```python
from build123d import *

# Parameters (mm, degrees)
SKETCH1_W           = 24
SKETCH1_H           = 3
BOSS_EXTRUDE1_DEPTH = 2
BOSS_EXTRUDE2_DEPTH = 3
BOSS_EXTRUDE3_DEPTH = 3
CUT_EXTRUDE1_REACH  = 23.383
SKETCH6_R           = 0.5
SKETCH9_W           = 3
SKETCH9_H           = 3
BOSS_EXTRUDE4_DEPTH = 0.5


with BuildPart() as part:
    # Sketch1 → Boss-Extrude1 (new body)
    with BuildSketch(Plane(origin=(0, 0, 0), x_dir=(1, 0, 0), z_dir=(0, 1, 0))):
        Rectangle(SKETCH1_W, SKETCH1_H)
    extrude(amount=BOSS_EXTRUDE1_DEPTH)

    # Sketch4 → Boss-Extrude2 (add)
    with BuildSketch(Plane(origin=(12, 0, 0), x_dir=(0, 0, -1), z_dir=(1, 0, 0))):
        Polygon((-11.5, 10), (-1.5, 0), (1.5, 0), (1.5, 2), (-0.5, 2), (-8.5, 10), align=None)
    extrude(amount=BOSS_EXTRUDE2_DEPTH)

    # Sketch5 → Boss-Extrude3 (add)
    with BuildSketch(Plane.ZY.offset(12)):
        Polygon((1.5, 0), (11.5, 10), (8.5, 10), (0.5, 2), (-1.5, 2), (-1.5, 0), align=None)
    extrude(amount=BOSS_EXTRUDE3_DEPTH)

    # Sketch6 → Cut-Extrude1 (cut, up to next)
    with BuildSketch(Plane.XZ, mode=Mode.PRIVATE) as cut_extrude1_sk1:
        with Locations(Location((-10, 0, 0), (0, 0, 270))):
            Circle(SKETCH6_R)
    cut_extrude1_tool1 = extrude(cut_extrude1_sk1.sketch, amount=-CUT_EXTRUDE1_REACH, mode=Mode.PRIVATE) & part.part
    # Sketch6 → Cut-Extrude1 (cut, up to next)
    with BuildSketch(Plane.XZ, mode=Mode.PRIVATE) as cut_extrude1_sk2:
        with Locations(Location((10, 0, 0), (0, 0, 270))):
            Circle(SKETCH6_R)
    cut_extrude1_tool2 = extrude(cut_extrude1_sk2.sketch, amount=-CUT_EXTRUDE1_REACH, mode=Mode.PRIVATE) & part.part
    add(cut_extrude1_tool1.solids().sort_by_distance((-10, 0, 0))[0], mode=Mode.SUBTRACT)
    add(cut_extrude1_tool2.solids().sort_by_distance((10, 0, 0))[0], mode=Mode.SUBTRACT)

    # Sketch9 → Boss-Extrude4 (add)
    with BuildSketch(Plane(origin=(0, 10, 0), x_dir=(1, 0, 0), z_dir=(0, 1, 0))):
        with Locations((-13.5, -10)):
            Rectangle(SKETCH9_W, SKETCH9_H)
        with Locations((13.5, -10)):
            Rectangle(SKETCH9_W, SKETCH9_H)
    extrude(amount=BOSS_EXTRUDE4_DEPTH)


solid = part.part
```
Input: part model. Units: mm. Frame: model coordinates. A direction names the side the tool comes from. Coordinates: 2 decimals unless noted, no trailing zeros. Loops run counter-clockwise (first coordinate to the right, second up) from the corner with the lowest first, then second, coordinate; pieces in that order, holes last. Notation, with made-up numbers: M 56,-30.75 L 114,-30.75 A27 cw 114,-8.75 Z; hole C 28,42 d4. An arc over 180 degrees is marked long. Use a Markdown table: item, result. Add a question column.
1) Section C-C, the plane z = 0. Return the cut outline in (x, y), plus the area to 3 significant figures.
2) Section B-B, the plane z = 4.75. Return the cut outline in (x, y), plus the area to 3 significant figures.
3) Draft query along X for faces 4 (the flat face through (0, 1, -1.5)), 5 (the flat face through (12, 6, 6)), 6 (the flat face through (-15, 5, 5)). Return one class per face: +X half, -X half, draft (parallel to the pull), parting line (faces both ways), or undercut.
4) Section A-A, the plane x = -10. Return the cut outline in (y, z).
5) Pin query (flat end, axial travel): P1, Ø0.9, axis at x = 3, z = 0.5, coming from the +Y side; P2, Ø1.6, axis at x = 2.5, y = 1, coming from the +Z side; P3, Ø3, axis at x = 0, z = 3.5, coming from the +Y side. Return the tip coordinate at first contact, or that it passes through.
6) Section D-D, the plane x = -0.5. Return the cut outline in (y, z).
7) Set-up query: faces 1 (the flat face through (0, 2, 0)), 2 (the flat face through (0, 1, 1.5)), 3 (the flat face through (15, 5, 5)). Return all of +Z, -Z, +X, -X, +Y, -Y with unobstructed straight access to the full face (end or side cutting, diameter ignored); none if empty.
8) Line query: L1, parallel to X at y = 0.85, z = 0; L2, parallel to X at y = 9.25, z = 8.25; L3, parallel to Y at x = -4.75, z = 0. Output: solid intervals per line, ascending. Write a range as from..to.
Answer below:
| question | item | result |
|---|---|---|
| 1 | outline | M -15,0 L -10.5,0 L -10.5,2 L -15,2 Z; M -9.5,0 L 9.5,0 L 9.5,2 L -9.5,2 Z; M 10.5,0 L 15,0 L 15,2 L 10.5,2 Z |
| 1 | area | 56.0 mm2 |
| 2 | outline | M -15,3.25 L -12,3.25 L -12,6.25 L -15,6.25 Z; M 12,3.25 L 15,3.25 L 15,6.25 L 12,6.25 Z |
| 2 | area | 18.0 mm2 |
| 3 | face 4 | draft |
| 3 | face 5 | undercut |
| 3 | face 6 | -X half |
| 4 | outline | M 0,-1.5 L 2,-1.5 L 2,-0.5 L 0,-0.5 Z; M 0,0.5 L 2,0.5 L 2,1.5 L 0,1.5 Z |
| 5 | P1 | y = 2 |
| 5 | P2 | z = 1.5 |
| 5 | P3 | through |
| 6 | outline | M 0,-1.5 L 2,-1.5 L 2,1.5 L 0,1.5 Z |
| 7 | face 1 | -Z, +Y |
| 7 | face 2 | +Z, +Y, -Y |
| 7 | face 3 | +Z, -Z, +X, +Y, -Y |
| 8 | L1 | -15..-10.5, -9.5..9.5, 10.5..15 |
| 8 | L2 | -15..-12, 12..15 |
| 8 | L3 | 0..2 |
